```python
from build123d import *

# Parameters (mm, degrees)
SKETCH001_R  = 45
PAD_DEPTH    = 1.12
SKETCH_W     = 8
SKETCH_H     = 70
PAD003_DEPTH = 3
SKETCH024_R  = 45
PAD006_DEPTH = 1


with BuildPart() as part:
    # Sketch001 → Pad (new body)
    with BuildSketch(Plane.XY):
        with BuildLine():
            Line((50, 64), (0, 64))
            ThreePointArc((0, 64), (-64.000064, 0), (0, -64))
            Line((50, -64), (0, -64))
            ThreePointArc((50, -64), (66.580186, -57.580186), (73, -41))
            Line((73, 41), (73, -41))
            ThreePointArc((73, 41), (66.580186, 57.580186), (50, 64))
        make_face()
        Circle(SKETCH001_R, mode=Mode.SUBTRACT)
    extrude(amount=-PAD_DEPTH)

    # Sketch → Pad003 (new body)
    with BuildSketch(Plane.XY):
        with Locations((69, 0)):
            Rectangle(SKETCH_W, SKETCH_H)
    extrude(amount=PAD003_DEPTH)

    # Sketch024 → Pad006 (new body)
    with BuildSketch(Plane.XY):
        with BuildLine():
            ThreePointArc((8.501021, 46.7331), (-47.5, 0), (8.501021, -46.7331))
            Line((8.501021, -46.7331), (73, -35))
            Line((73, 35), (73, -35))
            Line((8.501021, 46.7331), (73, 35))
        make_face()
        Circle(SKETCH024_R, mode=Mode.SUBTRACT)
    extrude(amount=PAD006_DEPTH)


solid = part.part
```
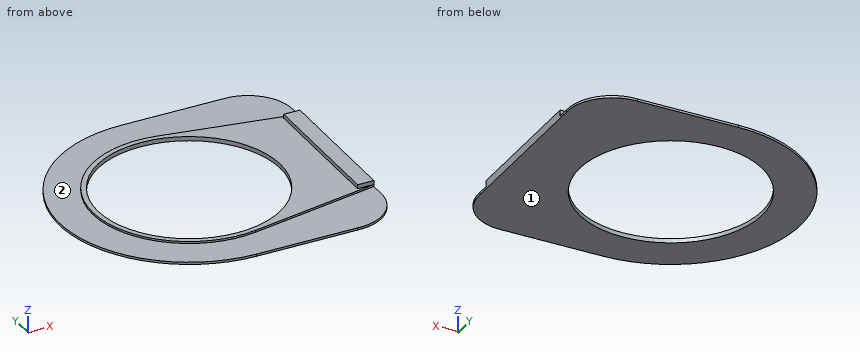
Source: CAD feature listing. Evaluate the final solid. Frame: model axes, mm. Face numbers are marked on the shaded views. A direction names the side the tool comes from. Coordinates: 2 decimals unless noted, no trailing zeros. Loops run counter-clockwise (first coordinate to the right, second up) from the corner with the lowest first, then second, coordinate; pieces in that order, holes last. Notation, with made-up numbers: (28.25, 5.5) -> (52.25, 5.5) arc R25 ccw to (52.25, 33.5) -> close; hole circle Ø1 at (12.25, -25.5). An arc over 180 degrees is marked (long way). One line per item, written item: value. Start each with the question number.
Q1. Section query B-B, the plane x = -22. Return the cut outline in (y, z), and give its area (3 significant figures).
Q2. Section query C-C, the plane z = 1.9. Return the cut outline in (x, y), and give its area (3 significant figures).
Q3. Contact query for flat-ended pins moving along their axis: P1, Ø2, axis at y = 40.5, z = 0.5, coming from the -X side; P2, Ø2, axis at y = 32.5, z = 0.5, coming from the +X side; P3, Ø10, axis at x = -8.5, y = 43.5, coming from the -Z side; P4, Ø1.6, axis at y = -9, z = 2.5, coming from the -X side. Output: stop coordinate, or through.
Q4. Line query: line 1 along Y through (x, z) = (0, 0.1); line 2 along X through (y, z) = (5, 1.05); line 3 along Z through (x, y) = (48, -37.5). Output: solid intervals per line, ascending.
Q5. Set-up query: the marked faces 1 and 2. Return all of +Z, -Z, +X, -X, +Y, -Y with unobstructed straight access to the full face (end or side cutting, diameter ignored); none if empty.
Q6. Section query A-A, the plane y = 0. Return the cut outline in (x, z), and give its area (3 significant figures).
Results:
1. outline: (-60.1, -1.12) -> (-39.26, -1.12) -> (-39.26, 1) -> (-42.1, 1) -> (-42.1, 0) -> (-60.1, 0) -> close; (39.26, -1.12) -> (60.1, -1.12) -> (60.1, 0) -> (42.1, 0) -> (42.1, 1) -> (39.26, 1) -> close
1. area: 52.4 mm^2
2. outline: (65, -35) -> (73, -35) -> (73, 35) -> (65, 35) -> close
2. area: 560 mm^2
3. P1: x = -50.25
3. P2: x = 73
3. P3: z = -1.12
3. P4: x = 65
4. line 1: -47.5 to -45, 45 to 47.5
4. line 2: 65 to 73
4. line 3: -1.12 to 1
5. face 1: -Z, +X, -X, +Y, -Y
5. face 2: +Z
6. outline: (-64, -1.12) -> (-45, -1.12) -> (-45, 1) -> (-47.5, 1) -> (-47.5, 0) -> (-64, 0) -> close; (45, -1.12) -> (73, -1.12) -> (73, 3) -> (65, 3) -> (65, 1) -> (45, 1) -> close
6. area: 99.1 mm^2
